from build123d import *

# Parameters (mm, degrees)
F1_DEPTH = 25
F3_R     = 5
F4_R     = 2.49999


# Not quite as in the source:
# - a fillet or chamfer is up to 0.001 mm smaller than in the source, because OpenCascade refuses the exact size


with BuildPart() as f1:
    # F0 (on Top) → F1 (new body)
    with BuildSketch(Plane.XY):
        Polygon((0, 25), (0, 0), (14.5, 0), (14.5, 20), (26.5, 20), (26.5, -20.958767963), (80.6644264157, -11.4081181913), (79.7961855273, -6.4840794262), (31.5, -15), (31.5, 25), align=None)
    extrude(amount=F1_DEPTH)

    # F3
    f3_edges = [f1.edges().sort_by_distance(p)[0] for p in [
        (26.5, -20.958768, 12.5),
        (31.5, -15, 12.5),
    ]]
    fillet(f3_edges, radius=F3_R)

    # F4 (radius 2.5 in the source; OpenCascade refuses exactly that, so slightly less here)
    f4_edges = [f1.edges().sort_by_distance(p)[0] for p in [
        (31.5, 25, 12.5),
        (79.796186, -6.484079, 12.5),
        (80.664426, -11.408118, 12.5),
        (14.5, 0, 12.5),
        (0, 0, 12.5),
        (0, 25, 12.5),
    ]]
    fillet(f4_edges, radius=F4_R)


solid = f1.part
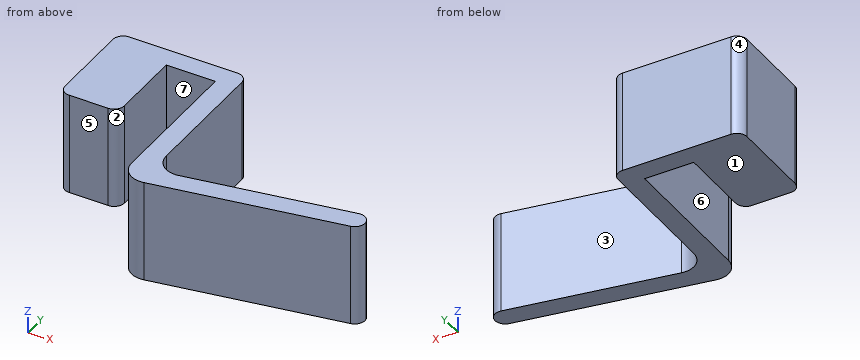
Check sheet for the modelled part. Datum: model origin and axes. Units: mm. Face numbers are marked on the shaded views. A direction names the side the tool comes from. Give positions to 0.01 mm unless a question says otherwise; leave off trailing zeros. Loops run counter-clockwise (first coordinate to the right, second up) from the corner with the lowest first, then second, coordinate; pieces in that order, holes last. Notation, with made-up numbers: M 12.5,-28.75 L 32.5,-28.75 A11 cw 32.5,-14.75 Z; hole C 45.25,72 d11. An arc over 180 degrees is marked long. Answer as a JSON object with one key per item and string values. Group by question number.
Q1. Access from +Z, -Z, +X, -X, +Y, -Y to the whole of each face (thin tool, end or side, straight path). Record for the marked faces 1, 2 and 3.
Q2. Cross-section at C-C on y = 1. Record the cut outline in (x, z).
Q3. Cross-section at D-D on x = 8. Record the cut outline in (y, z).
Q4. Release check for a two-part mould opening along X. For the marked faces 4, 5, 6 and 7 record: released by +X, released by -X, zero draft, split by the parting line, or undercut.
Q5. Cross-section at A-A on y = 16. Record the cut outline in (x, z).
Q6. Material ranges on line 1 along X through (y, z) = (8, 4); line 2 along X through (y, z) = (-4, 6.75); line 3 along Y through (x, z) = (15.5, 19.5), recorded low to high. Write a range as [from, to].
Q7. Go/stop test with flat-tipped pins: P1, Ø6, axis at x = 36.5, y = -10.5, coming from the +Z side; P2, Ø3, axis at y = -2, z = 15.5, coming from the +X side; P3, Ø2, axis at x = 36, z = 12, coming from the -Y side; P4, Ø5, axis at x = 28, z = 3, coming from the -Y side. Record where each tip stops, or that it passes through.
Evaluation:
{
 "1": {"face 1": "-Z, +X, -X, +Y, -Y", "face 2": "+Z, -Z, -Y", "face 3": "+Z, -Z, +Y"},
 "2": {"outline": "M 0.5,0 L 14,0 L 14,25 L 0.5,25 Z; M 26.5,0 L 31.5,0 L 31.5,25 L 26.5,25 Z"},
 "3": {"outline": "M 0,0 L 25,0 L 25,25 L 0,25 Z"},
 "4": {"face 4": "released by -X", "face 5": "zero draft", "face 6": "undercut", "face 7": "undercut"},
 "5": {"outline": "M 0,0 L 14.5,0 L 14.5,25 L 0,25 Z; M 26.5,0 L 31.5,0 L 31.5,25 L 26.5,25 Z"},
 "6": {"line 1": "x = [0, 14.5], [26.5, 31.5]", "line 2": "x = [26.5, 31.5]", "line 3": "y = [20, 25]"},
 "7": {"P1": "passes through", "P2": "stops at x = 31.5", "P3": "stops at y = -19.46", "P4": "stops at y = -19.9"}
}
